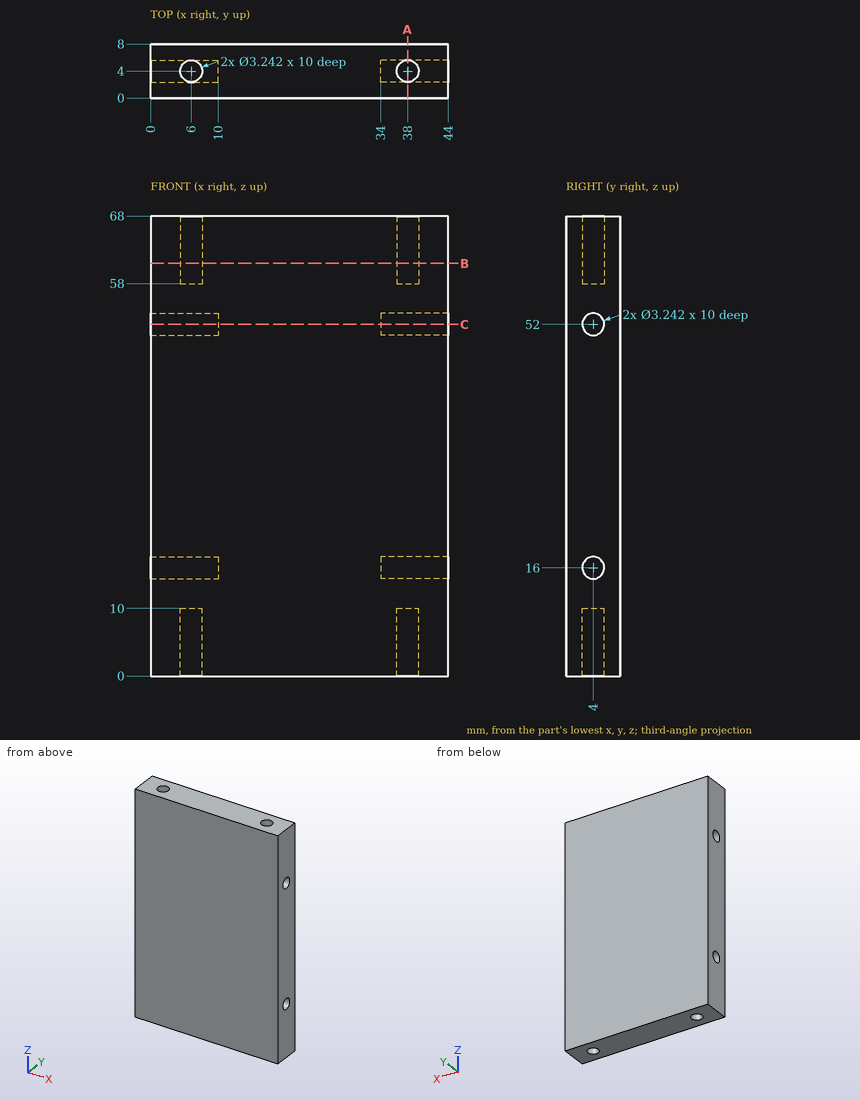
Study the drawing (mm; zero at the part's minimum x, y, z) and answer. Coordinates: 2 decimals unless noted, no trailing zeros. Write each loop counter-clockwise with the first axis right and the second up, starting at its lowest first coordinate (ties: lowest second). Pieces come first, ordered by that corner, then holes. Notation, with made-up numbers: (67, 87.5) - (71, 87.5) arc R25 ccw to (71, 99.5) - close; hole circle Ø6 at (88.25, 46). An arc over 180 degrees is marked (long way). One line per item, written item: value.
1) Each of these flat-tipped pins is pushed along its axis until it touches: pin 1 Ø1.6 at (y, z) = (4.5, 52) entering from -X; pin 2 Ø1 at (x, y) = (6, 4.5) entering from +Z; pin 3 Ø1 at (x, y) = (38.5, 4) entering from -Z. Where does it stop, or does it pass through?
Geometry check:
pin 1: stops at x = 10
pin 2: stops at z = 58
pin 3: stops at z = 10
2) Find section B-B (z = 61). Give the vertices of the cut face in (x, y).
Geometry check:
outline: (0, 0) - (44, 0) - (44, 8) - (0, 8) - close; hole circle Ø3.24 at (6, 4); hole circle Ø3.24 at (38, 4)
3) Find section C-C (z = 52). Give the vertices of the cut face in (x, y), and give its area (3 significant figures).
Geometry check:
outline: (0, 0) - (44, 0) - (44, 2.38) - (34, 2.38) - (34, 5.62) - (44, 5.62) - (44, 8) - (0, 8) - (0, 5.62) - (10, 5.62) - (10, 2.38) - (0, 2.38) - close
area: 287 mm2
4) Consider line 1 along Z through (x, y) = (5, 4); line 2 along Z through (x, y) = (2, 4); line 3 along X through (y, z) = (4, 3.5). Determine where each line is inside the solid, lowest interval first. Write a range as from..to.
Geometry check:
line 1: z = 10..14.38, 17.62..50.38, 53.62..58
line 2: z = 0..14.38, 17.62..50.38, 53.62..68
line 3: x = 0..4.38, 7.62..36.38, 39.62..44
5) Find section A-A (x = 38). Give the vertices of the cut face in (y, z), and give its area (3 significant figures).
Geometry check:
outline: (0, 0) - (2.38, 0) - (2.38, 10) - (5.62, 10) - (5.62, 0) - (8, 0) - (8, 68) - (5.62, 68) - (5.62, 58) - (2.38, 58) - (2.38, 68) - (0, 68) - close; hole circle Ø3.24 at (4, 16); hole circle Ø3.24 at (4, 52)
area: 463 mm2
